Verification items for the finished model (mm, model axes). Face numbers are marked on the shaded views. A direction names the side the tool comes from. Give positions to 0.01 mm unless a question says otherwise; leave off trailing zeros. Loops run counter-clockwise (first coordinate to the right, second up) from the corner with the lowest first, then second, coordinate; pieces in that order, holes last. Notation, with made-up numbers: M 11.5,11.25 L 53.5,11.25 A12 ccw 53.5,31.25 Z; hole C 17,76.25 d1. An arc over 180 degrees is marked long. Use CSV: the item, a comma, the result in double quotes.
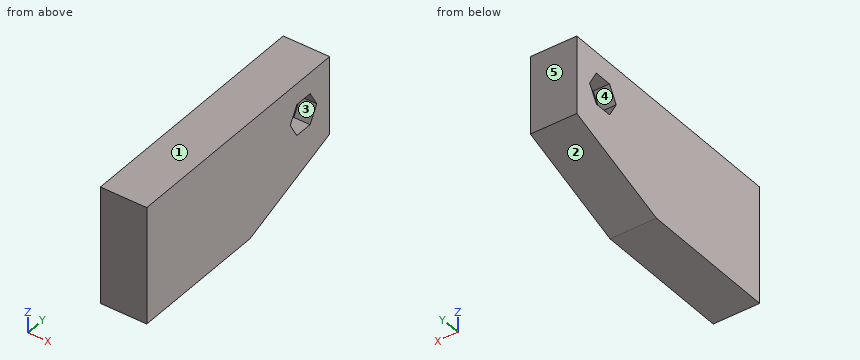
from build123d import *

# Parameters (mm, degrees)
SKETCH1_W           = 20
SKETCH1_H           = 107.436707244
BOSS_EXTRUDE1_DEPTH = 50.8
CUT_EXTRUDE2_DEPTH  = 7
CUT_EXTRUDE3_DEPTH  = 7
CUT_EXTRUDE4_REACH  = 147.208


with BuildPart() as part:
    # Sketch1 → Boss-Extrude1 (new body)
    with BuildSketch(Plane.XY):
        with Locations((94.748429341, -80.835326077)):
            Rectangle(SKETCH1_W, SKETCH1_H)
    extrude(amount=-BOSS_EXTRUDE1_DEPTH)

    # Sketch3 → Cut-Extrude2 (cut)
    with BuildSketch(Plane.ZY.offset(-84.748429341)):
        Polygon((-9.144783688, -38.547498147), (-15.914394935, -34.684550624), (-22.644611247, -38.615732175), (-22.605216312, -46.40986125), (-15.835605065, -50.272808774), (-9.105388753, -46.341627222), align=None)
    extrude(amount=-CUT_EXTRUDE2_DEPTH, mode=Mode.SUBTRACT)

    # Sketch4 → Cut-Extrude3 (cut)
    with BuildSketch(Plane(origin=(104.748429341, 0, 0), x_dir=(0, 0, -1), z_dir=(1, 0, 0))):
        Polygon((15.835605065, -50.272808774), (9.105388753, -46.341627222), (9.144783688, -38.547498147), (15.914394935, -34.684550624), (22.644611247, -38.615732175), (22.605216312, -46.40986125), align=None)
    extrude(amount=-CUT_EXTRUDE3_DEPTH, mode=Mode.SUBTRACT)

    # Sketch5 → Cut-Extrude4 (cut, up to next)
    with BuildSketch(Plane.ZY.offset(-84.748429341), mode=Mode.PRIVATE) as cut_extrude4_sk1:
        Polygon((-33.818744012, -27.116972455), (-50.8, -73.938366723), (-50.970000022, -27.115638049), align=None)
    cut_extrude4_tool1 = extrude(cut_extrude4_sk1.sketch, amount=-CUT_EXTRUDE4_REACH, mode=Mode.PRIVATE) & part.part
    add(cut_extrude4_tool1.solids().sort_by_distance((84.748429, -42.723659, -45.196248))[0], mode=Mode.SUBTRACT)


solid = part.part
(1) Mould release check, pull along Y, two halves, no side actions. Record for the marked faces 1, 2 and 3: released by +Y, released by -Y, zero draft, split by the parting line, or undercut.
Calculated:
face 1,"zero draft"
face 2,"released by +Y"
face 3,"undercut"
(2) Section check A-A on x = 90.5. Record the cut outline in (y, z).
Calculated:
outline,"M -134.55,-50.8 L -73.94,-50.8 L -27.12,-33.82 L -27.12,0 L -134.55,0 Z; hole M -50.27,-15.84 L -46.41,-22.61 L -38.62,-22.64 L -34.68,-15.91 L -38.55,-9.14 L -46.34,-9.11 Z"
(3) Section check D-D on z = -40. Record the cut outline in (x, y), plus the area to 3 significant figures.
Calculated:
outline,"M 84.75,-134.55 L 104.75,-134.55 L 104.75,-44.16 L 84.75,-44.16 Z"
area,"1,810 mm²"
(4) Tool access check on the marked faces 4 and 5. Record the directions out of +Z, -Z, +X, -X, +Y, -Y that give a thin tool (end or side, any length) a straight path to the whole face; none if there is none.
Calculated:
face 4,"-X"
face 5,"+Z, -Z, +X, -X, +Y"
(5) Section check C-C on y = -47.5. Record the cut outline in (x, z).
Calculated:
outline,"M 84.75,-41.21 L 104.75,-41.21 L 104.75,-20.69 L 97.75,-20.69 L 97.75,-11.09 L 104.75,-11.09 L 104.75,0 L 84.75,0 L 84.75,-11.09 L 91.75,-11.09 L 91.75,-20.69 L 84.75,-20.69 Z"
(6) Section check B-B on z = -21. Record the cut outline in (x, y).
Calculated:
outline,"M 84.75,-134.55 L 104.75,-134.55 L 104.75,-47.33 L 97.75,-47.33 L 97.75,-37.66 L 104.75,-37.66 L 104.75,-27.12 L 84.75,-27.12 L 84.75,-37.66 L 91.75,-37.66 L 91.75,-47.33 L 84.75,-47.33 Z"
(7) Scan lines: L1, parallel to X at y = -44, z = -21.5; L2, parallel to Y at x = 103.75, z = -12; L3, parallel to Y at x = 102.5, z = -18.5. Record each from-to range of solid material in increasing order. Write a range as from..to.
Calculated:
L1,"x = 91.75..97.75"
L2,"y = -134.55..-48.03, -36.92..-27.12"
L3,"y = -134.55..-48.75, -36.19..-27.12"
(8) Depth check by flat-ended pin: pin 1 Ø11 at (y, z) = (-41, -17) entering from +X; pin 2 Ø2 at (x, y) = (91, -52) entering from -Z. Enter the tip coordinate at first touch or a pass-through.
Calculated:
pin 1,"stops at x = 104.75"
pin 2,"stops at z = -43.21"
